from build123d import *

# Parameters (mm, degrees)
F0_R     = 8.5
F1_DEPTH = 4
F2_R     = 5
F3_DEPTH = 100


with BuildPart() as f1:
    # F0 (on Top) → F1 (new body)
    with BuildSketch(Plane.XY):
        Circle(F0_R)
    extrude(amount=F1_DEPTH)

    # F2 (on Top) → F3 (join)
    with BuildSketch(Plane.XY):
        Circle(F2_R)
    extrude(amount=F3_DEPTH)

    # F4 (on Right) → F5 (revolve)
    with BuildSketch(Plane.YZ):
        with BuildLine():
            Line((0, 104.0042367491), (0, 100))
            Line((0, 100), (5, 100))
            ThreePointArc((5, 100), (4.470554405, 102.2392282849), (2.9943426753, 104.0042367491))
            Line((2.9943426753, 104.0042367491), (0, 104.0042367491))
        make_face()
        with BuildLine():
            ThreePointArc((0, 105), (1.5777858306, 104.7445328403), (2.9943426753, 104.0042367491))
            ThreePointArc((2.9943426753, 104.0042367491), (2.1854582893, 106.243570465), (0, 107.1883887053))
            Line((0, 107.1883887053), (0, 105))
        make_face()
        with BuildLine():
            Line((0, 105), (0, 104.0042367491))
            Line((0, 104.0042367491), (2.9943426753, 104.0042367491))
            ThreePointArc((2.9943426753, 104.0042367491), (1.5777858306, 104.7445328403), (0, 105))
        make_face()
    revolve(axis=Axis((0, 0, 103.5941943526), (0, 0, -1)))


solid = f1.part
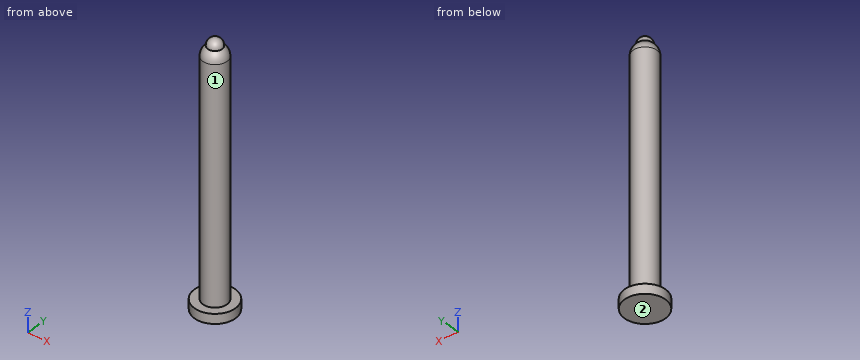
CAD build for the part. Positions are in the model's coordinates, mm. Face numbers are marked on the shaded views. A direction names the side the tool comes from. Round coordinates to 2 decimals unless told otherwise and drop trailing zeros. Loops run counter-clockwise (first coordinate to the right, second up) from the corner with the lowest first, then second, coordinate; pieces in that order, holes last. Notation, with made-up numbers: M 5,10 L 29,10 A25 ccw 29,23 Z; hole C -37,-14.5 d3. An arc over 180 degrees is marked long. One line per question, with ' | ' between items. Start each with the question number.
Item 1: Cut at A-A, the plane x = 4. Write the cut outline in (y, z), plus the area to 3 significant figures.
Item 2: Cut at C-C, the plane z = 32. Write the cut outline in (x, y).
Item 3: Pin check, flat tips, straight feed: pin 1 Ø5 at (x, y) = (0, -4) entering from +Z; pin 2 Ø1.5 at (y, z) = (-1.5, 65.5) entering from -X; pin 3 Ø8 at (y, z) = (-4, 28.5) entering from +X. Stop position of each tip, or through.
Item 4: Cut at B-B, the plane y = 0. Write the cut outline in (x, z).
Item 5: Which spindle directions (+Z, -Z, +X, -X, +Y, -Y) get a long thin tool onto all of the face, cutting with end or side? Do the marked faces 1 and 2. Say none if no direction does.
Item 6: Wall check: line 1 (Z direction, x = 7, y = 1); line 2 (Y direction, x = 0.25, z = 8); line 3 (X direction, y = 4, z = 10). Give the ranges that are in metal, low to high.
Responses:
1) outline: M -7.5,0 L 7.5,0 L 7.5,4 L 3,4 L 3,100 A3 ccw -3,100 L -3,4 L -7.5,4 Z | area: 650 mm²
2) outline: C 0,0 d10
3) pin 1: stops at z = 106.79 | pin 2: stops at x = -4.94 | pin 3: stops at x = 5
4) outline: M -8.5,0 L 8.5,0 L 8.5,4 L 5,4 L 5,100 A5 ccw 2.99,104 A3 ccw long -2.99,104 A5 ccw -5,100 L -5,4 L -8.5,4 Z
5) face 1: +Z | face 2: -Z, +X, -X, +Y, -Y
6) line 1: z = 0 to 4 | line 2: y = -4.99 to 4.99 | line 3: x = -3 to 3
